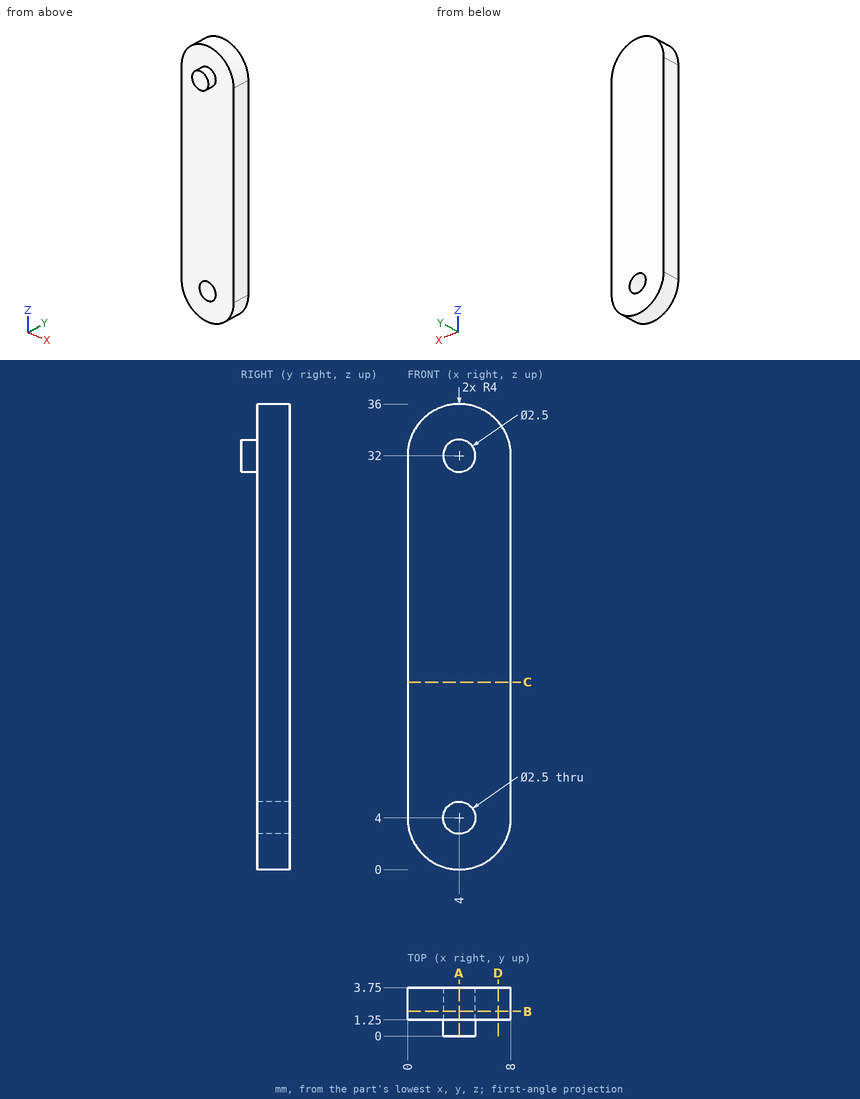
Geometry: see drawing. Coordinates: mm, zero at the bounding-box minimum. Give positions to 0.01 mm unless a question says otherwise; leave off trailing zeros. Write each loop counter-clockwise with the first axis right and the second up, starting at its lowest first coordinate (ties: lowest second). Pieces come first, ordered by that corner, then holes. Notation, with made-up numbers: (0.25, -34) -> (22.25, -34) arc R12 ccw to (22.25, -16) -> close; hole circle Ø6 at (3.5, 18). An arc over 180 degrees is marked (long way). Use one line per item in the form item = value. Start each with the question number.
1) Section query D-D on x = 7. Return the cut outline in (y, z).
2) Ray query, probe 1 along Z at (x, y) = (4, 2.9); probe 2 along X at (y, z) = (2.1, 4); probe 3 along Y at (x, z) = (2.5, 5). Return the intervals inside material, ascending. Write a range as from..to.
3) Section query B-B on y = 1.9. Return the cut outline in (x, z).
4) Pin query (flat end, axial travel): pin 1 (1 mm diameter, centred on x = 6, y = 1, fed in from +Z); pin 2 (2 mm diameter, centred on x = 2.5, y = 1.5, fed in from -Z). Return the tip coordinate at first contact, or that it passes through.
5) Section query A-A on x = 4. Return the cut outline in (y, z).
6) Section query C-C on z = 14.5. Return the cut outline in (x, y).
Outcome:
q1.outline = (1.25, 1.35) -> (3.75, 1.35) -> (3.75, 34.65) -> (1.25, 34.65) -> close
q2.probe_1 = 0..2.75, 5.25..36
q2.probe_2 = 0..2.75, 5.25..8
q2.probe_3 = 1.25..3.75
q3.outline = (0, 4) arc R4 ccw to (8, 4) -> (8, 32) arc R4 ccw to (0, 32) -> close; hole circle Ø2.5 at (4, 4)
q4.pin_1 = 35.68
q4.pin_2 = 0.03
q5.outline = (0, 30.75) -> (1.25, 30.75) -> (1.25, 5.25) -> (3.75, 5.25) -> (3.75, 36) -> (1.25, 36) -> (1.25, 33.25) -> (0, 33.25) -> close; (1.25, 0) -> (3.75, 0) -> (3.75, 2.75) -> (1.25, 2.75) -> close
q6.outline = (0, 1.25) -> (8, 1.25) -> (8, 3.75) -> (0, 3.75) -> close
